The model under review builds one solid part; all positions refer to its coordinate system, in mm. Coordinates: 2 decimals unless noted, no trailing zeros. Loops run counter-clockwise (first coordinate to the right, second up) from the corner with the lowest first, then second, coordinate; pieces in that order, holes last. Notation, with made-up numbers: M 75.25,-11.5 L 87.25,-11.5 A24 cw 87.25,23.5 Z; hole C -33,24 d9. An arc over 180 degrees is marked long. Return JSON: item names as keys, results as strings.
```python
from build123d import *

# Parameters (mm, degrees)
CROQUIS2_R              = 4
SALIENTE_EXTRUIR1_DEPTH = 13
CROQUIS3_R              = 25
CORTAR_EXTRUIR1_DEPTH   = 14
CROQUIS3_3_R            = 4
CORTAR_EXTRUIR2_DEPTH   = 14


with BuildPart() as part:
    # Croquis2 → Saliente-Extruir1 (new body)
    with BuildSketch(Plane.XY):
        with BuildLine():
            Line((-105, 160), (105, 160))
            ThreePointArc((105, 160), (112.071067812, 157.071067812), (115, 150))
            Line((115, 150), (115, -150))
            ThreePointArc((115, -150), (112.071067812, -157.071067812), (105, -160))
            Line((105, -160), (-105, -160))
            ThreePointArc((-105, -160), (-112.071067812, -157.071067812), (-115, -150))
            Line((-115, -150), (-115, 150))
            ThreePointArc((-115, 150), (-112.071067812, 157.071067812), (-105, 160))
        make_face()
        with Locations((-100, -145)):
            Circle(CROQUIS2_R, mode=Mode.SUBTRACT)
        with Locations((-100, 145)):
            Circle(CROQUIS2_R, mode=Mode.SUBTRACT)
        with Locations((100, -145)):
            Circle(CROQUIS2_R, mode=Mode.SUBTRACT)
        with Locations((100, 145)):
            Circle(CROQUIS2_R, mode=Mode.SUBTRACT)
    extrude(amount=SALIENTE_EXTRUIR1_DEPTH)

    # Croquis3 → Cortar-Extruir1 (cut, through all)
    with BuildSketch(Plane.XY.offset(13)):
        Circle(CROQUIS3_R)
    extrude(amount=-CORTAR_EXTRUIR1_DEPTH, mode=Mode.SUBTRACT)

    # Croquis3<3> → Cortar-Extruir2 (cut, through all)
    with BuildSketch(Plane.XY.offset(13)):
        with Locations((30, 0)):
            Circle(CROQUIS3_3_R)
        with Locations((0, 30)):
            Circle(CROQUIS3_3_R)
        with Locations((-30, 0)):
            Circle(CROQUIS3_3_R)
        with Locations((0, -30)):
            Circle(CROQUIS3_3_R)
    extrude(amount=-CORTAR_EXTRUIR2_DEPTH, mode=Mode.SUBTRACT)


solid = part.part
```
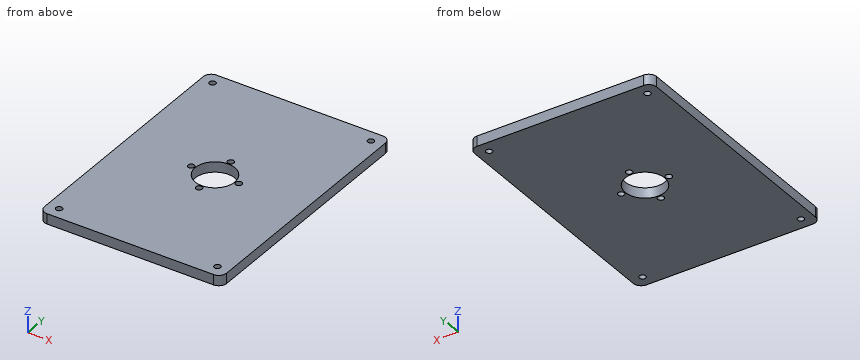
1. Add section D-D on x = 30. Give the boundary of the cut face in (y, z).
Check values:
{"outline": "M -160,0 L -4,0 L -4,13 L -160,13 Z; M 4,0 L 160,0 L 160,13 L 4,13 Z"}
2. Add section B-B on x = 100. Give the boundary of the cut face in (y, z), plus the area to 3 significant figures.
Check values:
{"outline": "M -160,0 L -149,0 L -149,13 L -160,13 Z; M -141,0 L 141,0 L 141,13 L -141,13 Z; M 149,0 L 160,0 L 160,13 L 149,13 Z", "area": "3,950 mm²"}
3. Insertion check: pin 1 Ø7 at (x, y) = (-100, -145) entering from +Z. The pin has a flat end and moves straight along its axis. Give the tip position at first contact, or say it passes through.
Check values:
{"pin 1": "through"}
4. Add section C-C on y = -30. Give the boundary of the cut face in (x, z), plus the area to 3 significant figures.
Check values:
{"outline": "M -115,0 L -4,0 L -4,13 L -115,13 Z; M 4,0 L 115,0 L 115,13 L 4,13 Z", "area": "2,890 mm²"}
5. To check wall thickness, follow line 1 (Y direction, x = 0, z = 3.75); line 2 (Y direction, x = 100, z = 7); line 3 (Y direction, x = 99, z = 4.75). State the ranges of each line that lie inside material, in increasing order.
Check values:
{"line 1": "-160 to -34, -26 to -25, 25 to 26, 34 to 160", "line 2": "-160 to -149, -141 to 141, 149 to 160", "line 3": "-160 to -148.87, -141.13 to 141.13, 148.87 to 160"}
6. Add section A-A on y = 145. Give the boundary of the cut face in (x, z), plus the area to 3 significant figures.
Check values:
{"outline": "M -115,0 L -104,0 L -104,13 L -115,13 Z; M -96,0 L 96,0 L 96,13 L -96,13 Z; M 104,0 L 115,0 L 115,13 L 104,13 Z", "area": "2,780 mm²"}
